Print and shaded views of the part. All mm, measured from the part's lowest x, y and z. Give positions to 0.01 mm unless a question says otherwise; leave off trailing zeros. Loops run counter-clockwise (first coordinate to the right, second up) from the corner with the lowest first, then second, coordinate; pieces in that order, holes last.
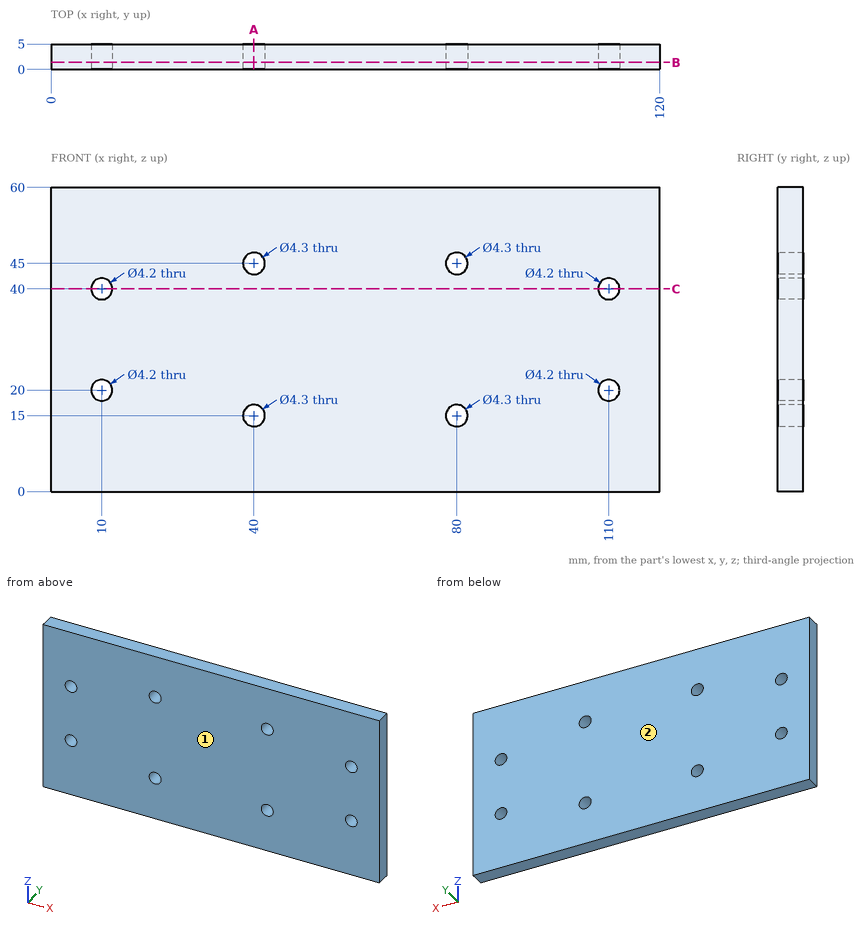
1. Probe line 1 along Z through (x, y) = (40, 3.4); line 2 along Z through (x, y) = (110, 1.35); line 3 along X through (y, z) = (3, 45). List the from-to ranges inside material, lowest first.
Responses:
line 1: z = 0 to 12.85, 17.15 to 42.85, 47.15 to 60
line 2: z = 0 to 17.9, 22.1 to 37.9, 42.1 to 60
line 3: x = 0 to 37.85, 42.15 to 77.85, 82.15 to 120
2. Saw through at A-A, the plane x = 40. List the corners of the cut face in (y, z).
Responses:
outline: (0, 0) - (5, 0) - (5, 12.85) - (0, 12.85) - close; (0, 17.15) - (5, 17.15) - (5, 42.85) - (0, 42.85) - close; (0, 47.15) - (5, 47.15) - (5, 60) - (0, 60) - close
3. Drop a flat-ended pin along its axis: pin 1 (4 mm diameter, centred on x = 10, z = 40, fed in from +Y). Give the stop position or say it passes through.
Responses:
pin 1: passes through
4. Pull direction Y, two halves, no side cores. Call the marked faces 1 and 2: released by +Y, released by -Y, zero draft, split by the parting line, or undercut.
Responses:
face 1: released by -Y
face 2: released by +Y
5. Saw through at B-B, the plane y = 1.4. Count the separate pieces of the cut face and the enclosed holes in it, and give its area (3 significant figures).
Responses:
separate pieces: 1
enclosed holes: 8
area: 7,090 mm2
6. Saw through at C-C, the plane z = 40. List the corners of the cut face in (x, y).
Responses:
outline: (0, 0) - (7.9, 0) - (7.9, 5) - (0, 5) - close; (12.1, 0) - (107.9, 0) - (107.9, 5) - (12.1, 5) - close; (112.1, 0) - (120, 0) - (120, 5) - (112.1, 5) - close
